Input: part model. Units: mm. Frame: model coordinates. Face numbers are marked on the shaded views. A direction names the side the tool comes from. Coordinates: 2 decimals unless noted, no trailing zeros. Loops run counter-clockwise (first coordinate to the right, second up) from the corner with the lowest first, then second, coordinate; pieces in that order, holes last. Notation, with made-up numbers: (3, 5.25) -> (38, 5.25) arc R20 ccw to (38, 11.25) -> close; hole circle Ø6 at (13.25, 24). An arc over 180 degrees is marked (long way). Answer as a JSON object with one key per item and string values.
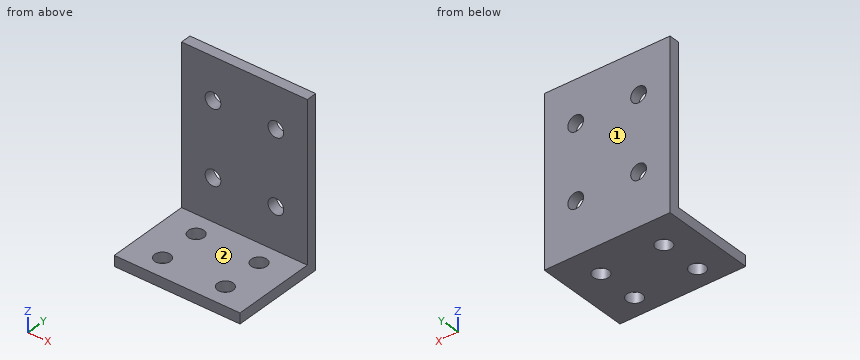
from build123d import *

# Parameters (mm, degrees)
F0_W     = 152.4
F0_H     = 203.2
F1_DEPTH = 12.7
F2_W     = 152.4
F2_H     = 12.7
F3_DEPTH = 101.6
F5_D     = 19.05
F5_DEPTH = 12.7
F7_D     = 19.05
F7_DEPTH = 12.7
F9_D     = 19.05
F9_DEPTH = 12.7


with BuildPart() as f1:
    # F0 (on Front) → F1 (new body)
    with BuildSketch(Plane.XZ):
        with Locations((76.2, 101.6)):
            Rectangle(F0_W, F0_H)
    extrude(amount=F1_DEPTH)

    # F2 (on face) → F3 (join)
    with BuildSketch(Plane.XZ.offset(12.7)):
        with Locations((76.2, 6.35)):
            Rectangle(F2_W, F2_H)
    extrude(amount=F3_DEPTH)

    # F5
    with Locations(Plane.XY.offset(12.7)):
        with Locations((38.1, -88.9)):
            Hole(F5_D / 2, depth=F5_DEPTH)

    # F7
    with Locations(Plane.XY.offset(12.7)):
        with Locations((38.1, -38.1), (114.3, -38.1), (114.3, -88.9)):
            Hole(F7_D / 2, depth=F7_DEPTH)

    # F9
    with Locations(Plane.XZ.offset(12.7)):
        with Locations((38.1, 152.4), (114.3, 152.4), (114.3, 63.5), (38.1, 63.5)):
            Hole(F9_D / 2, depth=F9_DEPTH)


solid = f1.part
1. Section query B-B (z = 63.5). Return loops of the section in (x, y) (3 decimals), plus the area to 3 significant figures.
Reply:
{"outline": "(0, -12.7) -> (28.575, -12.7) -> (28.575, 0) -> (0, 0) -> close; (47.625, -12.7) -> (104.775, -12.7) -> (104.775, 0) -> (47.625, 0) -> close; (123.825, -12.7) -> (152.4, -12.7) -> (152.4, 0) -> (123.825, 0) -> close", "area": "1,450 mm2"}
2. Line query: line 1 along Z through (x, y) = (38.1, -7.5) (3 decimals); line 2 along X through (y, z) = (-38, 8); line 3 along Y through (x, z) = (38.1, 4.5) (3 decimals). Output: solid intervals per line, ascending.
Reply:
{"line 1": "z = 0 to 53.975, 73.025 to 142.875, 161.925 to 203.2", "line 2": "x = 0 to 28.58, 47.62 to 104.78, 123.82 to 152.4", "line 3": "y = -114.3 to -98.425, -79.375 to -47.625, -28.575 to 0"}
3. Section query D-D (x = 36.5). Return loops of the section in (y, z).
Reply:
{"outline": "(-114.3, 0) -> (-98.29, 0) -> (-98.29, 12.7) -> (-114.3, 12.7) -> close; (-79.51, 0) -> (-47.49, 0) -> (-47.49, 12.7) -> (-79.51, 12.7) -> close; (-28.71, 0) -> (0, 0) -> (0, 54.11) -> (-12.7, 54.11) -> (-12.7, 12.7) -> (-28.71, 12.7) -> close; (-12.7, 72.89) -> (0, 72.89) -> (0, 143.01) -> (-12.7, 143.01) -> close; (-12.7, 161.79) -> (0, 161.79) -> (0, 203.2) -> (-12.7, 203.2) -> close"}
4. Section query A-A (y = -10). Return loops of the section in (x, z) (3 decimals).
Reply:
{"outline": "(0, 0) -> (152.4, 0) -> (152.4, 203.2) -> (0, 203.2) -> close; hole circle Ø19.05 at (38.1, 63.5); hole circle Ø19.05 at (38.1, 152.4); hole circle Ø19.05 at (114.3, 63.5); hole circle Ø19.05 at (114.3, 152.4)"}
5. Pin query (flat end, axial travel): P1, Ø25, axis at x = 38.1, y = -88.9, coming from the +Z side. Return the tip coordinate at first contact, or that it passes through.
Reply:
{"P1": "stops at z = 12.7"}
6. Section query C-C (y = -38.1). Return loops of the section in (x, z) (3 decimals), plus the area to 3 significant figures.
Reply:
{"outline": "(0, 0) -> (28.575, 0) -> (28.575, 12.7) -> (0, 12.7) -> close; (47.625, 0) -> (104.775, 0) -> (104.775, 12.7) -> (47.625, 12.7) -> close; (123.825, 0) -> (152.4, 0) -> (152.4, 12.7) -> (123.825, 12.7) -> close", "area": "1,450 mm2"}
7. Access query for the marked faces 1 and 2. Directions: +Z, -Z, +X, -X, +Y, -Y. A direction counts if a zero-diameter tool reaches every point of the face in a straight line with its end or side. Return the directions, or none.
Reply:
{"face 1": "+Z, -Z, +X, -X, +Y", "face 2": "+Z, +X, -X, -Y"}
